```python
from build123d import *

# Parameters (mm, degrees)
F0_W     = 75.603081
F0_H     = 55.037481
F1_DEPTH = 51.816
F2_R     = 5.08
F3_R     = 5.08


with BuildPart() as f1:
    # F0 (on Top) → F1 (new body)
    with BuildSketch(Plane.XY):
        with Locations((8.422104, -12.143501)):
            Rectangle(F0_W, F0_H)
        Polygon((-16.648348, -10.478666), (-7.246927, -10.478666), (25.462179, -10.478666), (25.462179, -14.591787), (-7.246927, -14.591787), (-12.339364, -14.591787), (-16.648348, -14.591787), (-16.648348, -11.262118), align=None, mode=Mode.SUBTRACT)
    extrude(amount=F1_DEPTH)

    # F2
    f2_edges = [f1.edges().sort_by_distance(p)[0] for p in [
        (4.406915, -14.591787, 51.816),
    ]]
    fillet(f2_edges, radius=F2_R)

    # F3
    f3_edges = [f1.edges().sort_by_distance(p)[0] for p in [
        (8.422104, 15.375239, 51.816),
        (8.422104, -39.662242, 51.816),
        (46.223644, -12.143502, 51.816),
        (-29.379437, -12.143502, 51.816),
        (4.406915, -10.478666, 51.816),
        (-29.379437, -39.662242, 25.908),
        (46.223644, -39.662242, 25.908),
        (8.422104, -39.662242, 0),
        (46.223644, 15.375239, 25.908),
        (-29.379437, 15.375239, 25.908),
    ]]
    fillet(f3_edges, radius=F3_R)


solid = f1.part
```
Could you check a few things on this model? Use its own coordinates, in mm. A direction names the side the tool comes from. Round coordinates to 2 decimals unless told otherwise and drop trailing zeros. Loops run counter-clockwise (first coordinate to the right, second up) from the corner with the lowest first, then second, coordinate; pieces in that order, holes last.
Q1. I want a section at C-C (z = 42.5). Write out the boundary of the cut face in (x, y).
Q2. I want a section at D-D (z = 4). Write out the boundary of the cut face in (x, y).
Q3. I want a section at A-A (x = 5.5). Write out the boundary of the cut face in (y, z).
Q4. On a 3-axis mill with a long thin cutter (end or side, diameter ignored), from which of +Z, -Z, +X, -X, +Y, -Y can I reach the whole of each face in a straight line? I mean faces 1 (the flat face through (8, -39.662, 26)), 2 (the flat face through (4, -10.479, 23)), 3 (the cylindrical face through (4.11, -16.04, 50.29)). Say none if no direction works.
Q5. Please list where these lines run through material, in increasing order: L1, parallel to Y at x = 14.5, z = 13; L2, parallel to X at y = -12, z = 26.5; L3, parallel to Y at x = 43.5, z = 30.
Q6. I want a section at B-B (y = -12.5). Write out the boundary of the cut face in (x, z), and give its area (3 significant figures).
Q7. Thinking about a two-plate mould opening in Y: for faces 4 (the flat face through (5, -14.592, 23)), 5 (the cylindrical face through (8.88, 13.927, 50.288)), 6 (the cylindrical face through (-27.93, -11.83, 50.29)), which applies, pulls with the +Y half, pulls with the -Y half, needs draft (parallel to the pull), parting line crosses it, or undercut?
Answer below:
1. outline: (-29.38, -34.58) arc R5.08 ccw to (-24.3, -39.66) - (41.14, -39.66) arc R5.08 ccw to (46.22, -34.58) - (46.22, 10.3) arc R5.08 ccw to (41.14, 15.38) - (-24.3, 15.38) arc R5.08 ccw to (-29.38, 10.3) - close; hole (-16.65, -14.59) - (25.46, -14.59) - (25.46, -10.48) - (-16.65, -10.48) - close
2. outline: (-29.38, -34.58) arc R5.08 ccw to (-25.38, -39.55) - (42.22, -39.55) arc R5.08 ccw to (46.22, -34.58) - (46.22, 10.3) arc R5.08 ccw to (41.14, 15.38) - (-24.3, 15.38) arc R5.08 ccw to (-29.38, 10.3) - close; hole (-16.65, -14.59) - (25.46, -14.59) - (25.46, -10.48) - (-16.65, -10.48) - close
3. outline: (-39.66, 5.08) arc R5.08 ccw to (-34.58, 0) - (-14.59, 0) - (-14.59, 46.74) arc R5.08 ccw to (-19.67, 51.82) - (-34.58, 51.82) arc R5.08 ccw to (-39.66, 46.74) - close; (-10.48, 0) - (15.38, 0) - (15.38, 46.74) arc R5.08 ccw to (10.3, 51.82) - (-5.4, 51.82) arc R5.08 ccw to (-10.48, 46.74) - close
4. face 1: +Z, -Z, +X, -X, -Y
4. face 2: +Z, -Z
4. face 3: +Z
5. L1: y = -39.66 to -14.59, -10.48 to 15.38
5. L2: x = -29.38 to -16.65, 25.46 to 46.22
5. L3: y = -39.08 to 14.8
6. outline: (-29.38, 0) - (-16.65, 0) - (-16.65, 51.82) - (-24.3, 51.82) arc R5.08 ccw to (-29.38, 46.74) - close; (25.46, 0) - (46.22, 0) - (46.22, 46.74) arc R5.08 ccw to (41.14, 51.82) - (25.46, 51.82) - close
6. area: 1,720 mm2
7. face 4: undercut
7. face 5: pulls with the +Y half
7. face 6: needs draft
